Source: CAD feature listing. Evaluate the final solid. Frame: model axes, mm. A direction names the side the tool comes from. Coordinates: 2 decimals unless noted, no trailing zeros. Write each loop counter-clockwise with the first axis right and the second up, starting at its lowest first coordinate (ties: lowest second). Pieces come first, ordered by that corner, then holes. Notation, with made-up numbers: M 39,81 L 64,81 A16 cw 64,99 Z; hole C 66.5,-11 d5. An arc over 180 degrees is marked long. Answer as CSV lines item,"result". Start each with the question number.
1. Line query: probe 1 along Y at (x, z) = (-6, 177.5); probe 2 along Y at (x, z) = (0, 85.5); probe 3 along Y at (x, z) = (-4.75, 170). Output: solid intervals per line, ascending. Write a range as [from, to].
2. Section A-A on y = 0. Return the cut outline in (x, z), plus the area to 3 significant figures.
3. Contact query for flat-ended pins moving along their axis: pin 1 Ø2 at (y, z) = (-3.5, 165.5) entering from +X; pin 2 Ø5 at (y, z) = (1, 148) entering from -X; pin 3 Ø5 at (y, z) = (-1, 112.5) entering from +X; pin 4 Ø3 at (x, y) = (0, 0) entering from +Z. Output: stop coordinate, or through.
4. Reachability of faces 5 (the face through (-7, -10, 108)), 6 (the face through (0, 4, 108)), 7 (the face through (4, 0, 108)) from +Z, -Z, +X, -X, +Y, -Y: full face, straight path, thin tool, end or side. Return the list, or none.
5. Mould query, pull axis X, two halves, no side actions, for faces 1 (the face through (10, -7, 108)), 2 (the face through (0, -4, 108)), 3 (the face through (-0.54, 2.44, 108.46)), 4 (the face through (-4, 0, 108)). Classes: pulls with the +X half, pulls with the -X half, needs draft (parallel to the pull), parting line crosses it, or undercut.
Autodesk Fusion 360 part; units mm, degrees
sketch "Sketch1" plane through (0, 0, 0) normal (0, 0, 1) x (1, 0, 0)
  circle A0 centre (0, 0) radius 2.5
  arc A1 (-10, -8.5) -> (-8.5, -10) centre (-8.5, -8.5) ccw
  arc A2 (8.5, -10) -> (10, -8.5) centre (8.5, -8.5) ccw
  arc A3 (10, 8.5) -> (8.5, 10) centre (8.5, 8.5) ccw
  arc A4 (-8.5, 10) -> (-10, 8.5) centre (-8.5, 8.5) ccw
  line L0 (-6.987, 5.3) -> (-8, 5.3)
  line L1 (6.987, -5.3) -> (8, -5.3)
  line L2 (8, 5.3) -> (6.987, 5.3)
  line L3 (-8, -5.3) -> (-6.987, -5.3)
  line L4 (-5.3, -8) -> (-5.3, -6.987)
  line L5 (-5.3, 6.987) -> (-5.3, 8)
  line L6 (5.3, 8) -> (5.3, 6.987)
  line L7 (5.3, -6.987) -> (5.3, -8)
  line L8 (2.313, -4) -> (-2.313, -4)
  line L9 (-4, -2.313) -> (-4, 2.313)
  line L10 (-2.313, 4) -> (2.313, 4)
  line L11 (4, 2.313) -> (4, -2.313)
  line L12 (6.2799, -5.0071) -> (4.2929, -3.0201)
  line L13 (5.0071, -6.2799) -> (3.0201, -4.2929)
  line L14 (-5.0071, -6.2799) -> (-3.0201, -4.2929)
  line L15 (-6.2799, -5.0071) -> (-4.2929, -3.0201)
  line L16 (-4.2929, 3.0201) -> (-6.2799, 5.0071)
  line L17 (-3.0201, 4.2929) -> (-5.0071, 6.2799)
  line L18 (3.0201, 4.2929) -> (5.0071, 6.2799)
  line L19 (4.2929, 3.0201) -> (6.2799, 5.0071)
  line L20 (0, -15) -> (0, 19) construction
  line L21 (-20, 0) -> (20, 0) construction
  line L22 (-10, -8.5) -> (-10, -4.75)
  line L23 (-10, 4.75) -> (-10, 8.5)
  line L24 (8.5, -10) -> (4.75, -10)
  line L25 (-4.75, -10) -> (-8.5, -10)
  line L26 (10, 8.5) -> (10, 4.75)
  line L27 (10, -4.75) -> (10, -8.5)
  line L28 (-8.5, 10) -> (-4.75, 10)
  line L29 (4.75, 10) -> (8.5, 10)
  line L30 (5.3, -8) -> (3.1, -8)
  line L31 (-3.1, -8) -> (-5.3, -8)
  line L32 (8, -5.3) -> (8, -3.1)
  line L33 (8, 3.1) -> (8, 5.3)
  line L34 (-5.3, 8) -> (-3.1, 8)
  line L35 (3.1, 8) -> (5.3, 8)
  line L36 (-8, 5.3) -> (-8, 3.1)
  line L37 (-8, -3.1) -> (-8, -5.3)
  line L38 (-4.75, -10) -> (-3.1, -8)
  line L39 (4.75, -10) -> (3.1, -8)
  line L40 (10, -4.75) -> (8, -3.1)
  line L41 (8, 3.1) -> (10, 4.75)
  line L42 (4.75, 10) -> (3.1, 8)
  line L43 (-4.75, 10) -> (-3.1, 8)
  line L44 (-10, 4.75) -> (-8, 3.1)
  line L45 (-10, -4.75) -> (-8, -3.1)
  arc A5 (-5.0071, -6.2799) -> (-5.3, -6.987) centre (-4.3, -6.987) ccw
  arc A6 (5.3, -6.987) -> (5.0071, -6.2799) centre (4.3, -6.987) ccw
  arc A7 (3.0201, -4.2929) -> (2.313, -4) centre (2.313, -5) ccw
  arc A8 (-2.313, -4) -> (-3.0201, -4.2929) centre (-2.313, -5) ccw
  arc A9 (-6.987, -5.3) -> (-6.2799, -5.0071) centre (-6.987, -4.3) ccw
  arc A10 (-4.2929, -3.0201) -> (-4, -2.313) centre (-5, -2.313) ccw
  arc A11 (-4, 2.313) -> (-4.2929, 3.0201) centre (-5, 2.313) ccw
  arc A12 (-6.2799, 5.0071) -> (-6.987, 5.3) centre (-6.987, 4.3) ccw
  arc A13 (6.2799, -5.0071) -> (6.987, -5.3) centre (6.987, -4.3) ccw
  arc A14 (4, -2.313) -> (4.2929, -3.0201) centre (5, -2.313) ccw
  arc A15 (4.2929, 3.0201) -> (4, 2.313) centre (5, 2.313) ccw
  arc A16 (6.987, 5.3) -> (6.2799, 5.0071) centre (6.987, 4.3) ccw
  arc A17 (5.0071, 6.2799) -> (5.3, 6.987) centre (4.3, 6.987) ccw
  arc A18 (2.313, 4) -> (3.0201, 4.2929) centre (2.313, 5) ccw
  arc A19 (-3.0201, 4.2929) -> (-2.313, 4) centre (-2.313, 5) ccw
  arc A20 (-5.3, 6.987) -> (-5.0071, 6.2799) centre (-4.3, 6.987) ccw
  dimension "d3" = 5
  dimension "d4" = 1.5
  dimension "d5" = 16
  dimension "d6" = 10.6
  dimension "d7" = 10.6
  dimension "d8" = 16
  dimension "d23" = 1
extrude "Extrude1" add sketch "Sketch1" along normal blind 149

Autodesk Fusion 360 part; units mm, degrees
sketch "Sketch1" plane through (0, 0, 0) normal (0, 0, 1) x (1, 0, 0)
  circle A0 centre (0, 0) radius 2.5
  arc A1 (-10, -8.5) -> (-8.5, -10) centre (-8.5, -8.5) ccw
  arc A2 (8.5, -10) -> (10, -8.5) centre (8.5, -8.5) ccw
  arc A3 (10, 8.5) -> (8.5, 10) centre (8.5, 8.5) ccw
  arc A4 (-8.5, 10) -> (-10, 8.5) centre (-8.5, 8.5) ccw
  line L0 (-6.987, 5.3) -> (-8, 5.3)
  line L1 (6.987, -5.3) -> (8, -5.3)
  line L2 (8, 5.3) -> (6.987, 5.3)
  line L3 (-8, -5.3) -> (-6.987, -5.3)
  line L4 (-5.3, -8) -> (-5.3, -6.987)
  line L5 (-5.3, 6.987) -> (-5.3, 8)
  line L6 (5.3, 8) -> (5.3, 6.987)
  line L7 (5.3, -6.987) -> (5.3, -8)
  line L8 (2.313, -4) -> (-2.313, -4)
  line L9 (-4, -2.313) -> (-4, 2.313)
  line L10 (-2.313, 4) -> (2.313, 4)
  line L11 (4, 2.313) -> (4, -2.313)
  line L12 (6.2799, -5.0071) -> (4.2929, -3.0201)
  line L13 (5.0071, -6.2799) -> (3.0201, -4.2929)
  line L14 (-5.0071, -6.2799) -> (-3.0201, -4.2929)
  line L15 (-6.2799, -5.0071) -> (-4.2929, -3.0201)
  line L16 (-4.2929, 3.0201) -> (-6.2799, 5.0071)
  line L17 (-3.0201, 4.2929) -> (-5.0071, 6.2799)
  line L18 (3.0201, 4.2929) -> (5.0071, 6.2799)
  line L19 (4.2929, 3.0201) -> (6.2799, 5.0071)
  line L20 (0, -15) -> (0, 19) construction
  line L21 (-20, 0) -> (20, 0) construction
  line L22 (-10, -8.5) -> (-10, -4.75)
  line L23 (-10, 4.75) -> (-10, 8.5)
  line L24 (8.5, -10) -> (4.75, -10)
  line L25 (-4.75, -10) -> (-8.5, -10)
  line L26 (10, 8.5) -> (10, 4.75)
  line L27 (10, -4.75) -> (10, -8.5)
  line L28 (-8.5, 10) -> (-4.75, 10)
  line L29 (4.75, 10) -> (8.5, 10)
  line L30 (5.3, -8) -> (3.1, -8)
  line L31 (-3.1, -8) -> (-5.3, -8)
  line L32 (8, -5.3) -> (8, -3.1)
  line L33 (8, 3.1) -> (8, 5.3)
  line L34 (-5.3, 8) -> (-3.1, 8)
  line L35 (3.1, 8) -> (5.3, 8)
  line L36 (-8, 5.3) -> (-8, 3.1)
  line L37 (-8, -3.1) -> (-8, -5.3)
  line L38 (-4.75, -10) -> (-3.1, -8)
  line L39 (4.75, -10) -> (3.1, -8)
  line L40 (10, -4.75) -> (8, -3.1)
  line L41 (8, 3.1) -> (10, 4.75)
  line L42 (4.75, 10) -> (3.1, 8)
  line L43 (-4.75, 10) -> (-3.1, 8)
  line L44 (-10, 4.75) -> (-8, 3.1)
  line L45 (-10, -4.75) -> (-8, -3.1)
  arc A5 (-5.0071, -6.2799) -> (-5.3, -6.987) centre (-4.3, -6.987) ccw
  arc A6 (5.3, -6.987) -> (5.0071, -6.2799) centre (4.3, -6.987) ccw
  arc A7 (3.0201, -4.2929) -> (2.313, -4) centre (2.313, -5) ccw
  arc A8 (-2.313, -4) -> (-3.0201, -4.2929) centre (-2.313, -5) ccw
  arc A9 (-6.987, -5.3) -> (-6.2799, -5.0071) centre (-6.987, -4.3) ccw
  arc A10 (-4.2929, -3.0201) -> (-4, -2.313) centre (-5, -2.313) ccw
  arc A11 (-4, 2.313) -> (-4.2929, 3.0201) centre (-5, 2.313) ccw
  arc A12 (-6.2799, 5.0071) -> (-6.987, 5.3) centre (-6.987, 4.3) ccw
  arc A13 (6.2799, -5.0071) -> (6.987, -5.3) centre (6.987, -4.3) ccw
  arc A14 (4, -2.313) -> (4.2929, -3.0201) centre (5, -2.313) ccw
  arc A15 (4.2929, 3.0201) -> (4, 2.313) centre (5, 2.313) ccw
  arc A16 (6.987, 5.3) -> (6.2799, 5.0071) centre (6.987, 4.3) ccw
  arc A17 (5.0071, 6.2799) -> (5.3, 6.987) centre (4.3, 6.987) ccw
  arc A18 (2.313, 4) -> (3.0201, 4.2929) centre (2.313, 5) ccw
  arc A19 (-3.0201, 4.2929) -> (-2.313, 4) centre (-2.313, 5) ccw
  arc A20 (-5.3, 6.987) -> (-5.0071, 6.2799) centre (-4.3, 6.987) ccw
  dimension "d3" = 5
  dimension "d4" = 1.5
  dimension "d5" = 16
  dimension "d6" = 10.6
  dimension "d7" = 10.6
  dimension "d8" = 16
  dimension "d23" = 1
extrude "Extrude1" add sketch "Sketch1" along normal blind 220
Values:
1,probe 1,"[-10, -4.73], [4.73, 10]"
1,probe 2,"[-4, -2.5], [2.5, 4]"
1,probe 3,"[-10, -8], [-6.02, -3.48], [3.48, 6.02], [8, 10]"
2,outline,"M -4,0 L -2.5,0 L -2.5,220 L -4,220 Z; M 2.5,0 L 4,0 L 4,220 L 2.5,220 Z"
2,area,"660 mm²"
3,pin 1,"x = 9.7"
3,pin 2,"x = -8.48"
3,pin 3,"x = 8.48"
3,pin 4,"through"
4,face 5,"+Z, -Z, +X, -X, -Y"
4,face 6,"+Z, -Z, +Y"
4,face 7,"+Z, -Z, +X"
5,face 1,"pulls with the +X half"
5,face 2,"undercut"
5,face 3,"undercut"
5,face 4,"pulls with the -X half"
